The model under review builds one solid part; all positions refer to its coordinate system, in mm. A direction names the side the tool comes from. Give positions to 0.01 mm unless a question says otherwise; leave off trailing zeros. Write each loop counter-clockwise with the first axis right and the second up, starting at its lowest first coordinate (ties: lowest second). Pieces come first, ordered by that corner, then holes. Notation, with made-up numbers: (-21, 4.25) -> (24, 4.25) arc R16 ccw to (24, 34.25) -> close; hole circle Ø8 at (4.25, 11.25). An arc over 180 degrees is marked (long way). Use CSV: the item, a comma, the result in double quotes.
```python
from build123d import *

# Parameters (mm, degrees)
F0_R     = 12.7
F1_DEPTH = 60.325
F2_DEPTH = 19.05
F3_W     = 41.275
F3_H     = 34.798
F4_DEPTH = 50.8
F5_W     = 55.2958
F5_H     = 22.3266
F6_DEPTH = 63.5
F7_R     = 6.35
F8_DEPTH = 127
F9_R     = 7.874
F10_R    = 5.08
F11_R    = 5.08


with BuildPart() as f1:
    # F0 (on Front) → F1 (new body)
    with BuildSketch(Plane.XZ):
        with BuildLine():
            Line((85.852, 0), (22.352, 0))
            ThreePointArc((22.352, 0), (-15.8052507731, 15.8052507731), (0, -22.352))
            Line((0, -22.352), (91.8464, -22.352))
            Line((91.8464, -22.352), (85.852, 0))
        make_face()
        Circle(F0_R, mode=Mode.SUBTRACT)
        Polygon((117.2464, 0), (85.852, 0), (91.8464, -22.352), (117.2464, -22.352), align=None)
        with BuildLine():
            ThreePointArc((131.0386, 34.798), (127.4644153616, 16.0823576341), (117.2464, 0))
            Line((117.2464, 0), (117.2464, -22.352))
            Line((117.2464, -22.352), (194.2084, -22.352))
            Line((194.2084, -22.352), (194.2084, 0))
            Line((194.2084, 0), (150.0886, 0))
            Line((150.0886, 0), (150.0886, 34.798))
            Line((150.0886, 34.798), (131.0386, 34.798))
        make_face()
    extrude(amount=-F1_DEPTH)

    # F0 (on Front) → F2 (cut)
    with BuildSketch(Plane.XZ):
        Polygon((117.2464, 0), (85.852, 0), (91.8464, -22.352), (117.2464, -22.352), align=None)
    extrude(amount=-F2_DEPTH, mode=Mode.SUBTRACT)

    # F3 (on face) → F4 (cut)
    with BuildSketch(Plane.YZ.offset(150.0886)):
        with Locations((39.6875, 17.399)):
            Rectangle(F3_W, F3_H)
    extrude(amount=-F4_DEPTH, mode=Mode.SUBTRACT)

    # F5 (on Top) → F6 (cut, symmetric)
    with BuildSketch(Plane.XY):
        with Locations((-5.2959, 30.1625)):
            Rectangle(F5_W, F5_H)
    extrude(amount=F6_DEPTH, both=True, mode=Mode.SUBTRACT)

    # F7 (on face) → F8 (cut)
    with BuildSketch(Plane.XY):
        with Locations((155.3464, 37.973)):
            Circle(F7_R)
    extrude(amount=-F8_DEPTH, mode=Mode.SUBTRACT)

    # F9
    f9_edges = [f1.edges().sort_by_distance(p)[0] for p in [
        (194.2084, 30.1625, 0),
    ]]
    fillet(f9_edges, radius=F9_R)

    # F10
    f10_edges = [f1.edges().sort_by_distance(p)[0] for p in [
        (150.0886, 9.525, 34.798),
    ]]
    fillet(f10_edges, radius=F10_R)

    # F11
    f11_edges = [f1.edges().sort_by_distance(p)[0] for p in [
        (22.352, 9.4996, 0),
        (22.352, 50.8254, 0),
    ]]
    fillet(f11_edges, radius=F11_R)


solid = f1.part
```
Q1. Machinability: for faces 1 (the flat face through (117.246, 9, -11)), 2 (the cylindrical face through (127.56, 9.39, 16.33)), 3 (the flat face through (88.8, 9.4, -11)), 4 (the flat face through (22.352, 30, -11)), 5 (the flat face through (150.089, 9, 15)), which of the approach directions +Z, -Z, +X, -X, +Y, -Y give a long, thin tool a straight path to every point of the face, cutting with its end or side? Answer none if there is none.
Derived:
face 1,"+Z, -Z, -Y"
face 2,"+Z, +Y, -Y"
face 3,"+Z, -Y"
face 4,"+Z, -Z, -X"
face 5,"+Z, +X, +Y, -Y"
Q2. Consider section A-A (y = 4). Write out the cut boundary in (x, z).
Derived:
outline,"(0, -22.35) -> (91.85, -22.35) -> (85.85, 0) -> (26.96, 0) arc R5.08 cw to (21.97, 4.14) arc R22.35 ccw (long way) to start; (117.25, -22.35) -> (194.21, -22.35) -> (194.21, -7.87) arc R7.87 ccw to (186.33, 0) -> (150.09, 0) -> (150.09, 29.72) arc R5.08 ccw to (145.01, 34.8) -> (131.04, 34.8) arc R50.8 cw to (117.25, 0) -> close; hole circle Ø25.4 at (0, 0)"
Q3. To check wall thickness, follow probe 1 along Z at (x, y) = (0, 53.5); probe 2 along Y at (x, z) = (-6.5, -16.5) (3 decimals); probe 3 along Z at (x, y) = (1, 58.5). State the ranges of each line that lie inside material, in increasing order.
Derived:
probe 1,"z = -22.35 to -12.7, 12.7 to 22.35"
probe 2,"y = 0 to 18.999, 41.326 to 60.325"
probe 3,"z = -22.35 to -12.66, 12.66 to 22.33"
Q4. Consider section B-B (x = 69). Write out the cut boundary in (y, z) (3 decimals).
Derived:
outline,"(0, -22.352) -> (60.325, -22.352) -> (60.325, 0) -> (0, 0) -> close"
Q5. Consider section C-C (x = 106.5). Write out the cut boundary in (y, z) (3 decimals), then the cut area to 3 significant figures.
Derived:
outline,"(19.05, -22.352) -> (60.325, -22.352) -> (60.325, 0) -> (19.05, 0) -> close"
area,"923 mm2"
Q6. The part is to be moulded in two halves that separate along Z. For faces 6 (the cylindrical face through (-2.75, 50.69, -12.4)), 7 (the cylindrical face through (-16.75, 50.69, 14.8)), 8 (the cylindrical face through (191.841, 30.585, -2.245)), 9 (the flat face through (13, 18.999, 0)), say which applies: pulls with the +Z half, pulls with the -Z half, needs draft (parallel to the pull), parting line crosses it, or undercut.
Derived:
face 6,"undercut"
face 7,"parting line crosses it"
face 8,"pulls with the +Z half"
face 9,"needs draft"
Q7. Insertion check: pin 1 (18 mm diameter, centred on y = 28.5, z = -10.5, fed in from -X); pin 2 (5.5 mm diameter, centred on y = 13, z = -12, fed in from -X); pin 3 (1 mm diameter, centred on x = 153.5, y = 26.5, fed in from +Z). Each pin has a flat end and moves straight along its axis. Give the tip position at first contact, or say it passes through.
Derived:
pin 1,"stops at x = 22.35"
pin 2,"stops at x = -20.35"
pin 3,"stops at z = 0"
